Geometry check sheet. Reference: the model listing, model coordinates, mm. A direction names the side the tool comes from. Give positions to 0.01 mm unless a question says otherwise; leave off trailing zeros. Order: outer loops, then holes, each group sorted by start corner. A loop starts at its lowest first (then second) coordinate and runs counter-clockwise, first axis right, second up. Notation, with made-up numbers: M 40.5,17.25 L 46.5,17.25 A33 ccw 46.5,46.25 Z; hole C 26.5,44 d10. An arc over 180 degrees is marked long. Answer as CSV lines item,"result".
from build123d import *

# Parameters (mm, degrees)
F1_W     = 4
F1_H     = 21.875
F3_W     = 25
F3_H     = 43.3012701892
F4_DEPTH = 75
F5_R     = 12.5
F6_DEPTH = 25
F7_R     = 3


# Not quite as in the source:
# - a feature names something its author has since deleted; it is built from what else it names


with BuildPart() as f2:
    # F1 (on Front) → F2 (revolve)
    with BuildSketch(Plane.XZ):
        with BuildLine():
            Line((0, 21.875), (0, 0))
            Line((0, 0), (145, 0))
            ThreePointArc((145, 0), (137.6776695297, 17.6776695297), (120, 25))
            Line((120, 25), (70, 25))
            Line((70, 25), (70, 37.5))
            Line((70, 37.5), (50, 37.5))
            Line((50, 37.5), (50, 20.75))
            Line((50, 20.75), (39.443375673, 20.75))
            Line((39.443375673, 20.75), (38, 20.75))
            Line((38, 20.75), (38, 23.25))
            Line((38, 23.25), (0, 23.25))
            Line((0, 23.25), (0, 21.875))
        make_face()
        Polygon((39.443375673, 20.75), (38, 23.25), (38, 20.75), align=None)
        with Locations((-2, 10.9375)):
            Rectangle(F1_W, F1_H)
    revolve(axis=Axis((72.5, 0, 0), (-1, 0, 0)))

    # F3 (on face) → F4 (cut)
    with BuildSketch(Plane.YZ.offset(70)):
        with Locations((-25, 0)):
            Rectangle(F3_W, F3_H)
        with Locations((25, 0)):
            Rectangle(F3_W, F3_H)
    extrude(amount=F4_DEPTH, mode=Mode.SUBTRACT)

    # F5 (on face) → F6 (cut, through all)
    with BuildSketch(Plane.XZ.offset(12.5)):
        with Locations((120, 0)):
            Circle(F5_R)
    extrude(amount=-F6_DEPTH, mode=Mode.SUBTRACT)

    # F7
    f7_edges = [f2.edges().sort_by_distance(p)[0] for p in [
        (70, -12.5, 0),
        (70, 12.5, 0),
        (70, 0, 25),
        (70, 0, -25),
    ]]
    fillet(f7_edges, radius=F7_R)


solid = f2.part
(1) Section check A-A on y = 0. Enter the section's corners in (x, z) (3 decimals), then the cut area to 3 significant figures.
The answers:
outline,"M -4,-21.875 L 0,-21.875 L 0,-23.25 L 38,-23.25 L 39.443,-20.75 L 50,-20.75 L 50,-37.5 L 70,-37.5 L 70,-28 A3 cw 73,-25 L 120,-25 A25 ccw 120,25 L 73,25 A3 cw 70,28 L 70,37.5 L 50,37.5 L 50,20.75 L 39.443,20.75 L 38,23.25 L 0,23.25 L 0,21.875 L -4,21.875 Z; hole C 120,0 d25"
area,"6,940 mm2"
(2) Draft check along X on faces 4 (the face through (59.86, 37.18, -4.88)), 5 (the face through (131.923, -0.175, 3.755)), 6 (the face through (70.9, -13.36, 0.33)). Enter one of: +X half, -X half, draft (parallel to the pull), parting line (faces both ways), or undercut.
The answers:
face 4,"draft"
face 5,"undercut"
face 6,"+X half"
(3) Section check D-D on z = 33. Enter the section's corners in (x, y).
The answers:
outline,"M 50,-17.81 L 70,-17.81 L 70,17.81 L 50,17.81 Z"
(4) Gauge pin test, flat ends, axial feed: P1, Ø3, axis at y = -11.5, z = -5, coming from the +X side; P2, Ø12, axis at x = 19.5, y = 4, coming from the +Z side; P3, Ø21.5, axis at x = 115.5, z = -9.5, coming from the +Y side. Record the tip position at first contact, or that the pin passes through.
The answers:
P1,"stops at x = 142.43"
P2,"stops at z = 23.25"
P3,"stops at y = 12.5"
(5) Material ranges on line 1 (X direction, y = -21, z = -17); line 2 (Y direction, x = 84.5, z = -9); line 3 (Z direction, x = 94.5, y = 1), recorded low to high.
The answers:
line 1,"x = 50 to 70"
line 2,"y = -12.5 to 12.5"
line 3,"z = -24.98 to 24.98"
(6) Tool access check on faces 1 (the face through (0, -9, 21)), 2 (the face through (96, 0, 25)), 3 (the face through (44.6, 6.2, 19.8)). Record the directions out of +Z, -Z, +X, -X, +Y, -Y that give a thin tool (end or side, any length) a straight path to the whole face; none if there is none.
The answers:
face 1,"-X"
face 2,"+Z, +X"
face 3,"none"
(7) Section check B-B on z = 0. Enter the section's corners in (x, y) (3 decimals).
The answers:
outline,"M -4,-21.875 L 0,-21.875 L 0,-23.25 L 38,-23.25 L 39.443,-20.75 L 50,-20.75 L 50,-37.5 L 70,-37.5 L 70,-15.5 A3 cw 73,-12.5 L 107.5,-12.5 L 107.5,12.5 L 73,12.5 A3 cw 70,15.5 L 70,37.5 L 50,37.5 L 50,20.75 L 39.443,20.75 L 38,23.25 L 0,23.25 L 0,21.875 L -4,21.875 Z; M 132.5,-12.5 L 141.651,-12.5 A25 ccw 141.651,12.5 L 132.5,12.5 Z"
(8) Section check C-C on x = 55. Enter the section's corners in (y, z).
The answers:
outline,"C 0,0 d75"
